```python
from build123d import *

# Parameters (mm, degrees)
F0_W      = 40
F0_H      = 22.5
F1_DEPTH  = 12
F3_DEPTH  = 40
F4_T      = -1.8
F6_E4_W   = 14.5
F6_E4_H   = 19.2
F7_DEPTH  = 3.6
F8_E5_W   = 14.5
F8_E5_H   = 19.2
F9_DEPTH  = 3.6
F10_W     = 5.25
F10_H     = 9
F11_DEPTH = 3.7
F12_W     = 5.25
F12_H     = 9
F13_DEPTH = 3.7
F14_W     = 1.5
F14_H     = 9
F15_DEPTH = 3.6
F16_W     = 1.5
F16_H     = 9
F17_DEPTH = 3.6
F18_W     = 7.75
F18_H     = 2.5
F19_DEPTH = 1.8
F20_W     = 7.75
F20_H     = 2.5
F21_DEPTH = 1.8
F23_DEPTH = 7.75
F25_DEPTH = 7.75
F27_DEPTH = 1.8
F29_DEPTH = 1.8
F30_R     = 2


with BuildPart() as f1:
    # F0 (on Top) → F1 (new body)
    with BuildSketch(Plane.XY):
        with Locations((-2.1441839635, 2.8779831225)):
            Rectangle(F0_W, F0_H)
    extrude(amount=F1_DEPTH)

    # F2 (on face) → F3 (cut)
    with BuildSketch(Plane.YZ.offset(17.8558160365)):
        Polygon((-8.3720168775, 12), (-8.3720168775, 0), (-5.3720168775, 12), align=None)
    extrude(amount=-F3_DEPTH, mode=Mode.SUBTRACT)

    # F4
    f4_openings = [f1.faces().sort_by_distance(p)[0] for p in [
        (-2.144184, 2.877983, 0),
    ]]
    offset(amount=F4_T, openings=f4_openings)

    # F6_E4 (on explicit) → F7 (join)
    with BuildSketch(Plane(origin=(-10.3441839635, -3.966619346, 10.2), x_dir=(0, 1, 0), z_dir=(-1, 0, 0))):
        with Locations((7.25, 9.6)):
            Rectangle(F6_E4_W, F6_E4_H)
    extrude(amount=F7_DEPTH)

    # F8_E5 (on explicit) → F9 (join)
    with BuildSketch(Plane(origin=(6.0558160365, -3.966619346, 10.2), x_dir=(0, 1, 0), z_dir=(-1, 0, 0))):
        with Locations((7.25, 9.6)):
            Rectangle(F8_E5_W, F8_E5_H)
    extrude(amount=-F9_DEPTH)

    # F10 (on face) → F11 (cut)
    with BuildSketch(Plane.YZ.offset(9.6558160365)):
        with Locations((-1.341619346, -4.5)):
            Rectangle(F10_W, F10_H)
    extrude(amount=-F11_DEPTH, mode=Mode.SUBTRACT)

    # F12 (on face) → F13 (cut)
    with BuildSketch(Plane(origin=(-13.9441839635, 0, 0), x_dir=(0, -1, 0), z_dir=(-1, 0, 0))):
        with Locations((1.341619346, -4.5)):
            Rectangle(F12_W, F12_H)
    extrude(amount=-F13_DEPTH, mode=Mode.SUBTRACT)

    # F14 (on face) → F15 (cut)
    with BuildSketch(Plane.YZ.offset(9.6558160365)):
        with Locations((9.783380654, -4.5)):
            Rectangle(F14_W, F14_H)
    extrude(amount=-F15_DEPTH, mode=Mode.SUBTRACT)

    # F16 (on face) → F17 (cut)
    with BuildSketch(Plane(origin=(-13.9441839635, 0, 0), x_dir=(0, -1, 0), z_dir=(-1, 0, 0))):
        with Locations((-9.783380654, -4.5)):
            Rectangle(F16_W, F16_H)
    extrude(amount=-F17_DEPTH, mode=Mode.SUBTRACT)

    # F18 (on face) → F19 (cut)
    with BuildSketch(Plane(origin=(-13.9441839635, 0, 0), x_dir=(0, -1, 0), z_dir=(-1, 0, 0))):
        with Locations((-5.158380654, -1.25)):
            Rectangle(F18_W, F18_H)
    extrude(amount=-F19_DEPTH, mode=Mode.SUBTRACT)

    # F20 (on face) → F21 (cut)
    with BuildSketch(Plane.YZ.offset(9.6558160365)):
        with Locations((5.158380654, -1.25)):
            Rectangle(F20_W, F20_H)
    extrude(amount=-F21_DEPTH, mode=Mode.SUBTRACT)

    # F22 (on face) → F23 (cut)
    with BuildSketch(Plane(origin=(0, 9.033380654, 0), x_dir=(-1, 0, 0), z_dir=(0, 1, 0))):
        Polygon((-6.0558160365, -9), (-9.6558160365, -2.5), (-9.6558160365, -9), align=None)
    extrude(amount=-F23_DEPTH, mode=Mode.SUBTRACT)

    # F24 (on face) → F25 (cut)
    with BuildSketch(Plane(origin=(0, 9.033380654, 0), x_dir=(-1, 0, 0), z_dir=(0, 1, 0))):
        Polygon((13.9441839635, -9), (13.9441839635, -2.5), (10.3441839635, -9), align=None)
    extrude(amount=-F25_DEPTH, mode=Mode.SUBTRACT)

    # F26 (on face) → F27 (cut)
    with BuildSketch(Plane(origin=(-22.1441839635, 0, 0), x_dir=(0, -1, 0), z_dir=(-1, 0, 0))):
        with BuildLine():
            Line((-0.1815545511, 0), (-0.1815545511, 6.4285714286))
            ThreePointArc((-0.1815545511, 6.4285714286), (-3.6815545511, 2.9285714286), (-7.1815545511, 6.4285714286))
            Line((-7.1815545511, 6.4285714286), (-7.1815545511, 0))
            Line((-7.1815545511, 0), (-0.1815545511, 0))
        make_face()
        with BuildLine():
            ThreePointArc((-7.1815545511, 6.4285714286), (-3.6815545511, 2.9285714286), (-0.1815545511, 6.4285714286))
            ThreePointArc((-0.1815545511, 6.4285714286), (-3.6815545511, 9.9285714286), (-7.1815545511, 6.4285714286))
        make_face()
    extrude(amount=-F27_DEPTH, mode=Mode.SUBTRACT)

    # F28 (on face) → F29 (cut)
    with BuildSketch(Plane.YZ.offset(17.8558160365)):
        with BuildLine():
            ThreePointArc((0.1815545511, 6.4285714286), (3.6815545511, 2.9285714286), (7.1815545511, 6.4285714286))
            ThreePointArc((7.1815545511, 6.4285714286), (3.6815545511, 9.9285714286), (0.1815545511, 6.4285714286))
        make_face()
        with BuildLine():
            Line((7.1815545511, 0), (7.1815545511, 6.4285714286))
            ThreePointArc((7.1815545511, 6.4285714286), (3.6815545511, 2.9285714286), (0.1815545511, 6.4285714286))
            Line((0.1815545511, 6.4285714286), (0.1815545511, 0))
            Line((0.1815545511, 0), (7.1815545511, 0))
        make_face()
    extrude(amount=-F29_DEPTH, mode=Mode.SUBTRACT)

    # F30
    f30_edges = [f1.edges().sort_by_distance(p)[0] for p in [
        (17.855816, -6.872017, 6),
        (17.855816, 14.127983, 6),
        (17.855816, 4.377983, 12),
        (-22.144184, -6.872017, 6),
        (-22.144184, 14.127983, 6),
        (-22.144184, 4.377983, 12),
        (-2.144184, -5.372017, 12),
        (-2.144184, 14.127983, 12),
    ]]
    fillet(f30_edges, radius=F30_R)


solid = f1.part
```
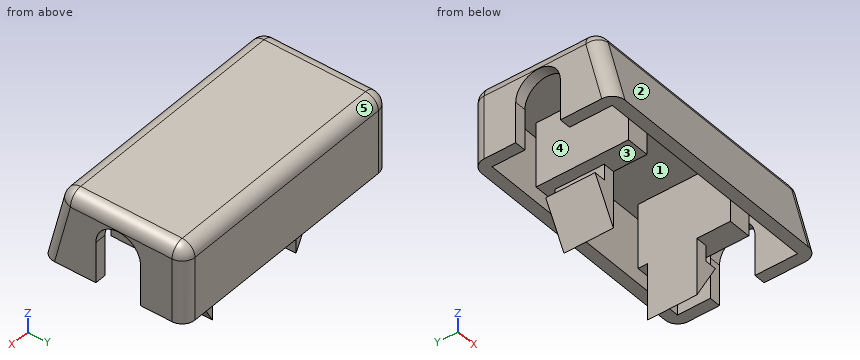
The listing builds one solid part. Answer for the finished solid, in the listing's coordinates (mm). Face numbers are marked on the shaded views. A direction names the side the tool comes from. Round coordinates to 2 decimals unless told otherwise and drop trailing zeros. Order: outer loops, then holes, each group sorted by start corner. A loop starts at its lowest first (then second) coordinate and runs counter-clockwise, first axis right, second up. Notation, with made-up numbers: (-30.5, -12) -> (-8.5, -12) arc R5 ccw to (-8.5, -4) -> close; hole circle Ø3 at (30, 42). An arc over 180 degrees is marked (long way). Answer as CSV lines item,"result".
Q1. A cutting plane is placed at C-C on x = 9. Determine the outline of the cut face in (y, z), plus the area to 3 significant figures.
Computed values:
outline,"(-8.37, 0) -> (-6.52, 0) -> (-3.97, 10.2) -> (-3.97, 0) -> (10.53, 0) -> (10.53, 10.2) -> (12.33, 10.2) -> (12.33, 0) -> (14.13, 0) -> (14.13, 10) arc R2 ccw to (12.13, 12) -> (-3.81, 12) arc R2 ccw to (-5.75, 10.49) -> close; (1.28, -3.68) -> (9.03, -3.68) -> (9.03, -2.5) -> (1.28, -2.5) -> close"
area,"229 mm^2"
Q2. A cutting plane is placed at D-D on x = -3. Determine the outline of the cut face in (y, z).
Computed values:
outline,"(-8.37, 0) -> (-6.52, 0) -> (-3.97, 10.2) -> (12.33, 10.2) -> (12.33, 0) -> (14.13, 0) -> (14.13, 10) arc R2 ccw to (12.13, 12) -> (-3.81, 12) arc R2 ccw to (-5.75, 10.49) -> close"
Q3. Consider line 1 (X direction, y = 4.5, z = 8.25); line 2 (Z direction, x = -16, y = 4.5); line 3 (Y direction, x = 11.5, z = 5). Determine where each line is inside the solid, lowest interval first. Write a range as from..to.
Computed values:
line 1,"x = -13.94..-10.34, 6.06..9.66"
line 2,"z = 10.2..12"
line 3,"y = -7.12..-5.27, 12.33..14.13"
Q4. A cutting plane is placed at A-A on z = -0.75. Determine the outline of the cut face in (x, y), plus the area to 3 significant figures.
Computed values:
outline,"(-12.14, 1.28) -> (-10.34, 1.28) -> (-10.34, 9.03) -> (-12.14, 9.03) -> close; (6.06, 1.28) -> (7.86, 1.28) -> (7.86, 9.03) -> (6.06, 9.03) -> close"
area,"27.9 mm^2"
Q5. A cutting plane is placed at B-B on y = -3. Determine the outline of the cut face in (x, z), plus the area to 3 significant figures.
Computed values:
outline,"(-22.14, 0) -> (-20.34, 0) -> (-20.34, 10.2) -> (-13.94, 10.2) -> (-13.94, 0) -> (-10.34, 0) -> (-10.34, 10.2) -> (6.06, 10.2) -> (6.06, 0) -> (9.66, 0) -> (9.66, 10.2) -> (16.06, 10.2) -> (16.06, 0) -> (17.86, 0) -> (17.86, 10) arc R2 ccw to (15.86, 12) -> (-20.14, 12) arc R2 ccw to (-22.14, 10) -> close"
area,"180 mm^2"
Q6. For a pull along Y with two mould halves and no side action, classify the marked faces 1, 2 and 3 as +Y half, -Y half, draft (parallel to the pull), parting line (faces both ways), or undercut.
Computed values:
face 1,"undercut"
face 2,"-Y half"
face 3,"draft"
Q7. Given pin 1 (1.8 mm diameter, centred on x = -11.5, y = 5, fed in from -Z); pin 2 (5 mm diameter, centred on y = 4, z = 3.5, fed in from +X); pin 3 (1.1 mm diameter, centred on x = 8, y = 4.5, fed in from -Z), each flat-ended and moving along its own axis, determine where each tip first touches the part or whether it passes through.
Computed values:
pin 1,"stops at z = -8.54"
pin 2,"stops at x = 9.66"
pin 3,"stops at z = -6.48"
Q8. Which of the six approach directions +Z, -Z, +X, -X, +Y, -Y give full straight-line access (tool end or side, diameter ignored) to the marked faces 4 and 5?
Computed values:
face 4,"-Z"
face 5,"+Z, +X, -X, +Y"
